Verification items for the finished model (mm, model axes). A direction names the side the tool comes from. Round coordinates to 2 decimals unless told otherwise and drop trailing zeros. Write each loop counter-clockwise with the first axis right and the second up, starting at its lowest first coordinate (ties: lowest second). Pieces come first, ordered by that corner, then holes. Notation, with made-up numbers: M 49,16 L 57,16 A8 ccw 57,22 Z; hole C -21,84 d4. An arc over 180 degrees is marked long. One line per question, with ' | ' between items.
from build123d import *

# Parameters (mm, degrees)
F1_DEPTH     = 10.2
F2_R         = 14.25
F3_DEPTH     = 7
F4_W         = 4.4
F4_H         = 30
F5_DEPTH     = 8.5
F7_DEPTH     = 25
F9_T1_DEPTH  = 42.5
F9_T4_ANGLE  = 180
F9_T6_ANGLE  = 180
F9_T10_DEPTH = 32.5676095837
F9_S11_R     = 14.25
F9_T12_DEPTH = 18


# Not quite as in the source:
# - a fillet or chamfer that OpenCascade refuses, or shapes differently, is made with other operations: its cross-section is extruded or revolved along the edge and cut away or added


with BuildPart() as f1:
    # F0 (on Top) → F1 (new body)
    with BuildSketch(Plane.XY):
        with BuildLine():
            Line((-17.5, 20), (-17.5, -20))
            Line((-17.5, -20), (17.5, -20))
            Line((17.5, -20), (17.5, 20))
            ThreePointArc((17.5, 20), (0, 2.5), (-17.5, 20))
        make_face()
        with BuildLine():
            Line((17.5, 20), (-17.5, 20))
            ThreePointArc((-17.5, 20), (0, 2.5), (17.5, 20))
        make_face()
        with BuildLine():
            ThreePointArc((17.5, 20), (0, 37.5), (-17.5, 20))
            Line((-17.5, 20), (17.5, 20))
        make_face()
    extrude(amount=-F1_DEPTH)


with BuildPart() as f3:
    # F2 (on Top) → F3 (new body)
    with BuildSketch(Plane.XY):
        with Locations((0, 20)):
            Circle(F2_R)
    extrude(amount=-F3_DEPTH)


with BuildPart() as f5:
    # F4 (on face) → F5 (new body)
    with BuildSketch(Plane(origin=(0, 0, -10.2), x_dir=(1, 0, 0), z_dir=(0, 0, -1))):
        with Locations((0, 5)):
            Rectangle(F4_W, F4_H)
    extrude(amount=-F5_DEPTH)


with BuildPart() as f7:
    # F6 (on face) → F7 (new body)
    with BuildSketch(Plane(origin=(0, 0, -10.2), x_dir=(1, 0, 0), z_dir=(0, 0, -1))):
        with BuildLine():
            Line((-13.7838047919, -16.3848616264), (13.7838047919, -16.3848616264))
            ThreePointArc((13.7838047919, -16.3848616264), (0, -5.75), (-13.7838047919, -16.3848616264))
        make_face()
    extrude(amount=-F7_DEPTH)


with BuildPart() as f1_1:
    add(f1.part)

    # F8: cut F7, F5, F3
    add(f7.part, mode=Mode.SUBTRACT)
    add(f5.part, mode=Mode.SUBTRACT)
    add(f3.part, mode=Mode.SUBTRACT)

    # F9: fillet of radius 1 on 3 edges, made by hand

    # F9_s2 → F9_t1 (cut)
    with BuildSketch(Plane.XZ.offset(-20)):
        with BuildLine():
            ThreePointArc((16.5, -10.2), (17.2071067812, -9.9071067812), (17.5, -9.2))
            Line((17.5, -9.2), (17.5, -10.2))
            Line((17.5, -10.2), (16.5, -10.2))
        make_face()
        with BuildLine():
            ThreePointArc((-17.5, -9.2), (-17.2071067812, -9.9071067812), (-16.5, -10.2))
            Line((-16.5, -10.2), (-17.5, -10.2))
            Line((-17.5, -10.2), (-17.5, -9.2))
        make_face()
        with BuildLine():
            ThreePointArc((16.5, 0), (17.2071067812, -0.2928932188), (17.5, -1))
            Line((17.5, -1), (17.5, 0))
            Line((17.5, 0), (16.5, 0))
        make_face()
        with BuildLine():
            ThreePointArc((-17.5, -1), (-17.2071067812, -0.2928932188), (-16.5, 0))
            Line((-16.5, 0), (-17.5, 0))
            Line((-17.5, 0), (-17.5, -1))
        make_face()
    extrude(amount=F9_T1_DEPTH, mode=Mode.SUBTRACT)

    # F9_s3 → F9_t4 (revolve, cut)
    with BuildSketch(Plane.XZ.offset(-20)):
        with BuildLine():
            ThreePointArc((17.5, -1), (17.2071067812, -0.2928932188), (16.5, 0))
            Line((16.5, 0), (17.5, 0))
            Line((17.5, 0), (17.5, -1))
        make_face()
    revolve(axis=Axis((0, 20, 0), (0, 0, 1)), revolution_arc=F9_T4_ANGLE, mode=Mode.SUBTRACT)

    # F9_s5 → F9_t6 (revolve, cut)
    with BuildSketch(Plane.XZ.offset(-20)):
        with BuildLine():
            ThreePointArc((17.5, -9.2), (17.2071067812, -9.9071067812), (16.5, -10.2))
            Line((16.5, -10.2), (17.5, -10.2))
            Line((17.5, -10.2), (17.5, -9.2))
        make_face()
    revolve(axis=Axis((0, 20, -10.2), (0, 0, 1)), revolution_arc=F9_T6_ANGLE, mode=Mode.SUBTRACT)


with BuildPart() as f9_tool8:
    # F9_s9 → F9_t10 (new body)
    with BuildSketch(Plane.YZ.offset(-16.2838047919)):
        with BuildLine():
            ThreePointArc((16.3848616264, -8), (16.6777548452, -7.2928932188), (17.3848616264, -7))
            Line((17.3848616264, -7), (16.3848616264, -7))
            Line((16.3848616264, -7), (16.3848616264, -8))
        make_face()
    extrude(amount=F9_T10_DEPTH)

    # F9_s11 → F9_t12 (intersect, symmetric)
    with BuildSketch(Plane.XY.offset(-7.5)):
        with Locations((0, 20)):
            Circle(F9_S11_R)
    extrude(amount=F9_T12_DEPTH, both=True, mode=Mode.INTERSECT)


with BuildPart() as f1_2:
    add(f1_1.part)

    # F9_t7: cut F9_tool8
    add(f9_tool8.part, mode=Mode.SUBTRACT)


solid = f1_2.part
1. Section check B-B, the plane z = -4. Record the cut outline in (x, y).
Results:
outline: M -17.5,-20 L -2.2,-20 L -2.2,5.92 A14.25 cw long 2.2,5.92 L 2.2,-20 L 17.5,-20 L 17.5,20 A17.5 ccw -17.5,20 Z
2. Section check C-C, the plane y = -10. Record the cut outline in (x, z).
Results:
outline: M -17.5,-9.2 A1 ccw -16.5,-10.2 L -2.2,-10.2 L -2.2,-1.7 L 2.2,-1.7 L 2.2,-10.2 L 16.5,-10.2 A1 ccw 17.5,-9.2 L 17.5,-1 A1 ccw 16.5,0 L -16.5,0 A1 ccw -17.5,-1 Z
3. Section check A-A, the plane x = 0. Record the cut outline in (y, z), then the cut area to 3 significant figures.
Results:
outline: M -20,-1.7 L 5.75,-1.7 L 5.75,0 L -20,0 Z; M 16.38,-10.2 L 36.5,-10.2 A1 ccw 37.5,-9.2 L 37.5,-1 A1 ccw 36.5,0 L 34.25,0 L 34.25,-7 L 17.38,-7 A1 ccw 16.38,-8 Z | area: 133 mm2
4. Thickness scan on line 1 (X direction, y = -8, z = -3.75); line 2 (X direction, y = 20, z = -2.5); line 3 (Y direction, x = 0, z = -4.25). Record the ranges inside material, lowest first.
Results:
line 1: x = -17.5 to -2.2, 2.2 to 17.5 | line 2: x = -17.5 to -14.25, 14.25 to 17.5 | line 3: y = 34.25 to 37.5
5. Go/stop test with flat-tipped pins: P1, Ø1.5, axis at y = 24.5, z = -9, coming from the -X side; P2, Ø4, axis at x = 10.5, z = -8, coming from the +Y side; P3, Ø13.5, axis at x = 0.5, y = 22.5, coming from the +Z side; P4, Ø3.5, axis at x = -0.5, y = -8, coming from the -Z side. Record where each tip stops, or that it passes through.
Results:
P1: stops at x = -17.09 | P2: stops at y = 35.3 | P3: stops at z = -7 | P4: stops at z = -10.2
6. Tool access check on faces 5 (the face through (2.2, -7, -6)), 6 (the face through (0, 16.385, -9)), 7 (the face through (0, 24, -7)). Record the directions out of +Z, -Z, +X, -X, +Y, -Y that give a thin tool (end or side, any length) a straight path to the whole face; none if there is none.
Results:
face 5: -Z, -Y | face 6: +Z, -Z | face 7: +Z
7. Mould release check, pull along X, two halves, no side actions. Record for faces 1 (the face through (-17.5, 0, -5)), 2 (the face through (-2.2, -7, -6)), 3 (the face through (0, -7, -1.7)), 4 (the face through (17.5, 0, -5)): pulls with the +X half, pulls with the -X half, needs draft (parallel to the pull), parting line crosses it, or undercut.
Results:
face 1: pulls with the -X half | face 2: undercut | face 3: undercut | face 4: pulls with the +X half
